from build123d import *

# Parameters (mm, degrees)
BOSS_EXTRU_1_DEPTH       = 44
ESQUISSE2_R              = 4.5
ENL_V_MAT_EXTRU_1_DEPTH  = 96
ESQUISSE6_R              = 2.75
ENL_V_MAT_EXTRU_2_DEPTH  = 96.0000001
ESQUISSE7_R              = 4.75
ENL_V_MAT_EXTRU_3_DEPTH  = 24
ESQUISSE8_R              = 2.75
ENL_V_MAT_EXTRU_4_DEPTH  = 96.0000001
ESQUISSE9_R              = 4.75
ENL_V_MAT_EXTRU_5_DEPTH  = 24
ESQUISSE10_R             = 2.75
ENL_V_MAT_EXTRU_6_DEPTH  = 96.0000001
ESQUISSE11_R             = 4.75
ENL_V_MAT_EXTRU_8_DEPTH  = 24
ESQUISSE13_R             = 4.75
ENL_V_MAT_EXTRU_11_DEPTH = 24
TROU_TARAUD_M51_D        = 4.2
CONG_1_R                 = 10


with BuildPart() as part:
    # Esquisse1 → Boss.-Extru.1 (new body)
    with BuildSketch(Plane.XY):
        with BuildLine():
            Line((-252.5, 75), (-252.5, 68.266055554))
            ThreePointArc((-252.5, 68.266055554), (-156.243343573, 16.179149841), (-50, -10.102813546))
            Line((-50, -10.102813546), (-50, -20))
            Line((-50, -20), (50, -20))
            Line((50, -20), (50, -10.102813546))
            ThreePointArc((50, -10.102813546), (156.243343573, 16.179149841), (252.5, 68.266055554))
            Line((252.5, 68.266055554), (252.5, 75))
            Line((252.5, 75), (239.5, 75))
            ThreePointArc((239.5, 75), (0, 0), (-239.5, 75))
            Line((-239.5, 75), (-252.5, 75))
        make_face()
    extrude(amount=BOSS_EXTRU_1_DEPTH)

    # Esquisse2 → Enlèv. mat.-Extru.1 (cut, through all)
    with BuildSketch(Plane.XZ.offset(20)):
        with Locations(Location((0, 22, 0), (0, 0, 270))):  # turned: the seam where the file's is
            Circle(ESQUISSE2_R)
    extrude(amount=-ENL_V_MAT_EXTRU_1_DEPTH, mode=Mode.SUBTRACT)

    # Esquisse6 → Enlèv. mat.-Extru.2 (cut, through all)
    with BuildSketch(Plane(origin=(0, 75, 0), x_dir=(1, 0, 0), z_dir=(0, 1, 0))):
        with Locations(Location((246, -8, 0), (0, 0, 270))):  # turned: the seam where the file's is
            Circle(ESQUISSE6_R)
    extrude(amount=-ENL_V_MAT_EXTRU_2_DEPTH, mode=Mode.SUBTRACT)

    # Esquisse7 → Enlèv. mat.-Extru.3 (cut)
    with BuildSketch(Plane(origin=(0, 45, 0), x_dir=(-1, 0, 0), z_dir=(0, 1, 0))):
        with Locations(Location((-246, 8, 0), (0, 0, 270))):  # turned: the seam where the file's is
            Circle(ESQUISSE7_R)
    extrude(amount=ENL_V_MAT_EXTRU_3_DEPTH, mode=Mode.SUBTRACT)

    # Esquisse8 → Enlèv. mat.-Extru.4 (cut, through all)
    with BuildSketch(Plane(origin=(0, 75, 0), x_dir=(1, 0, 0), z_dir=(0, 1, 0))):
        with Locations(Location((246, -36, 0), (0, 0, 270))):  # turned: the seam where the file's is
            Circle(ESQUISSE8_R)
    extrude(amount=-ENL_V_MAT_EXTRU_4_DEPTH, mode=Mode.SUBTRACT)

    # Esquisse9 → Enlèv. mat.-Extru.5 (cut)
    with BuildSketch(Plane(origin=(0, 45, 0), x_dir=(-1, 0, 0), z_dir=(0, 1, 0))):
        with Locations(Location((-246, 36, 0), (0, 0, 270))):  # turned: the seam where the file's is
            Circle(ESQUISSE9_R)
    extrude(amount=ENL_V_MAT_EXTRU_5_DEPTH, mode=Mode.SUBTRACT)

    # Esquisse10 → Enlèv. mat.-Extru.6 (cut, through all)
    with BuildSketch(Plane(origin=(0, 75, 0), x_dir=(1, 0, 0), z_dir=(0, 1, 0))):
        with Locations(Location((-246, -8, 0), (0, 0, 270))):  # turned: the seam where the file's is
            Circle(ESQUISSE10_R)
        with Locations(Location((-246, -36, 0), (0, 0, 270))):  # turned: the seam where the file's is
            Circle(ESQUISSE10_R)
    extrude(amount=-ENL_V_MAT_EXTRU_6_DEPTH, mode=Mode.SUBTRACT)

    # Esquisse11 → Enlèv. mat.-Extru.8 (cut)
    with BuildSketch(Plane(origin=(0, 45, 0), x_dir=(-1, 0, 0), z_dir=(0, 1, 0))):
        with Locations(Location((246, 8, 0), (0, 0, 270))):  # turned: the seam where the file's is
            Circle(ESQUISSE11_R)
    extrude(amount=ENL_V_MAT_EXTRU_8_DEPTH, mode=Mode.SUBTRACT)

    # Esquisse13 → Enlèv. mat.-Extru.11 (cut)
    with BuildSketch(Plane(origin=(0, 45, 0), x_dir=(-1, 0, 0), z_dir=(0, 1, 0))):
        with Locations(Location((245.795073353, 35.637141441, 0), (0, 0, 270))):  # turned: the seam where the file's is
            Circle(ESQUISSE13_R)
    extrude(amount=ENL_V_MAT_EXTRU_11_DEPTH, mode=Mode.SUBTRACT)

    # Trou taraudé M51 (through all)
    with Locations(Plane(origin=(0, 0, 0), x_dir=(-1, 0, 0), z_dir=(0, 0, -1))):
        with Locations((0, -10)):
            Hole(TROU_TARAUD_M51_D / 2)

    # Congé1
    cong_1_edges = [part.edges().sort_by_distance(p)[0] for p in [
        (-50, -10.102813546, 22),
        (50, -10.102813546, 22),
    ]]
    fillet(cong_1_edges, radius=CONG_1_R)


solid = part.part
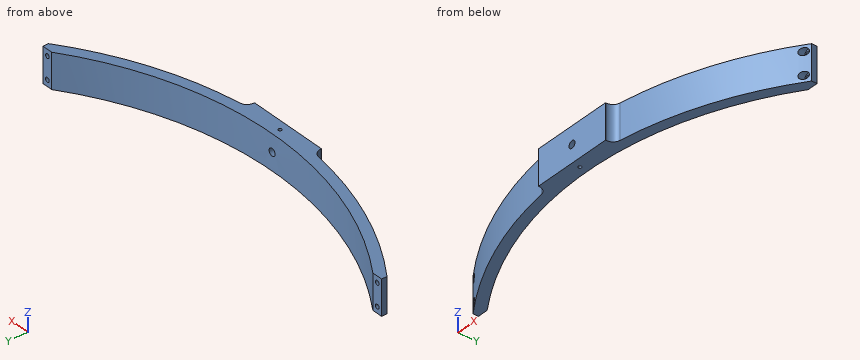
Design review of the part built by this model. Coordinates are the model's own, in mm. Round coordinates to 2 decimals unless told otherwise and drop trailing zeros. Loops run counter-clockwise (first coordinate to the right, second up) from the corner with the lowest first, then second, coordinate; pieces in that order, holes last. Notation, with made-up numbers: (48, 34.25) - (98, 34.25) arc R11 cw to (98, 54.25) - close; hole circle Ø4 at (15.5, 61). An arc over 180 degrees is marked (long way). One line per item, written item: value. Start each with the question number.
1) Consider section A-A on y = 18. Give the boundary of the cut face in (x, z), then the cut area to 3 significant figures.
2) Insertion check: pin 1 Ø1.5 at (y, z) = (35, 17) entering from -X; pin 2 Ø1.5 at (x, z) = (-184.5, 28.5) entering from -Y; pin 3 Ø1.2 at (y, z) = (-19.5, 21) entering from +X. Each pin has a flat end and moves straight along its axis. Give the tip position at first contact, or say it passes through.
3) To check wall thickness, follow L1, parallel to Z at x = -246, y = 66; L2, parallel to Y at x = 0, z = 34.25; L3, parallel to X at y = 64, z = 29.5. State the ranges of each line that lie inside material, in increasing order. Write a range as from..to.
4) Consider section B-B on x = 127. Give the boundary of the cut face in (y, z), then the cut area to 3 significant figures.
5) Consider section C-C on x = 195. Give the boundary of the cut face in (y, z), then the cut area to 3 significant figures.
Reported:
1. outline: (-160.87, 0) - (-121.62, 0) - (-121.62, 44) - (-160.87, 44) - close; (121.62, 0) - (160.87, 0) - (160.87, 44) - (121.62, 44) - close
1. area: 3,450 mm^2
2. pin 1: stops at x = -199.58
2. pin 2: stops at y = 27.93
2. pin 3: stops at x = 50
3. L1: z = 0..3.25, 12.75..30.89, 40.38..44
3. L2: y = -20..-12.1, -7.9..0
3. L3: x = -246.45..-222.83, 222.83..246.45
4. outline: (6.05, 0) - (19.67, 0) - (19.67, 44) - (6.05, 44) - close
4. area: 599 mm^2
5. outline: (33.41, 0) - (48.02, 0) - (48.02, 44) - (33.41, 44) - close
5. area: 643 mm^2
